Can you work these out from the model? Positions are in its coordinate system, mm. A direction names the side the tool comes from. Round coordinates to 2 decimals unless told otherwise and drop trailing zeros. Write each loop counter-clockwise with the first axis right and the second up, starting at its lowest first coordinate (ties: lowest second). Pieces come first, ordered by that corner, then holes. Notation, with made-up numbers: M -16.75,-35 L 5.25,-35 A17 ccw 5.25,-20 Z; hole C 34,65 d11. An arc over 180 degrees is marked long. Answer in a Markdown table with one row per item. Add a question column.
(1) If I drill on probe 1 along Z at (x, y) = (-1.25, 12.5); probe 2 along Y at (x, z) = (7.5, 1.7); probe 3 along X at (y, z) = (11.25, 166), over which ranges is the centre line in solid material (lowest first)?
(2) I'm going to push flat-ended pins straight in: pin 1 (2.5 mm diameter, centred on x = 16.5, z = 139.5, fed in from -Y); pin 2 (2 mm diameter, centred on y = 12.4, z = 100, fed in from +X); pin 3 (6.5 mm diameter, centred on x = 10, y = 7, fed in from +Z); pin 4 (4 mm diameter, centred on x = 3.5, y = 17, fed in from +Z). Where does each tip first touch, or does it pass through?
(3) If we mould it in two halves opening along X, with no side actions, what happens to faces 6 (the face through (9.885, -1.846, 1.521)), 7 (the face through (18, 10, 114)), 8 (the face through (7, 6, 3)), 9 (the face through (7, 19.403, 116))? For each: released by +X, released by -X, zero draft, split by the parting line, or undercut.
(4) Suppose I cut it at A-A, the plane y = 7.25. Write out the boundary of the cut face in (x, z).
(5) Suppose I cut it at B-B, the plane z = 135. Write out the boundary of the cut face in (x, y).
(6) For faces 1 (the face through (-1, 11, 8)), 2 (the face through (9, 20, 224)), 3 (the face through (7.17, 20.88, 220.48)), 4 (the face through (16, 11, 8)), 5 (the face through (0, 8, 114)), which set-ups out of +Z, -Z, +X, -X, +Y, -Y let a thin tool reach every point of the face, with its end or its side?
from build123d import *

# Parameters (mm, degrees)
F1_DEPTH  = 15
F2_W      = 3
F2_H      = 216
F3_DEPTH  = 25
F4_R      = 2.5
F5_DEPTH  = 3
F6_W      = 1
F6_H      = 0.5
F7_DEPTH  = 3
F8_R      = 1
F9_R      = 2.5
F9_R_2    = 1.2
F10_DEPTH = 3
F11_R     = 1.2
F12_DEPTH = 34.2
F13_DEPTH = 3
F14_R     = 2


with BuildPart() as f1:
    # F0 (on Right) → F1 (new body)
    with BuildSketch(Plane.YZ):
        Polygon((-7.5968508422, 3), (-7.5968508422, 0), (22.4031491578, 0), (22.4031491578, 224), (19.4031491578, 224), (19.4031491578, 3), align=None)
    extrude(amount=F1_DEPTH)

    # F2 (on face) → F3 (join)
    with BuildSketch(Plane(origin=(0, 22.4031491578, 0), x_dir=(-1, 0, 0), z_dir=(0, 1, 0))):
        with Locations((1.5, 116)):
            Rectangle(F2_W, F2_H)
        with Locations((-16.5, 116)):
            Rectangle(F2_W, F2_H)
    extrude(amount=-F3_DEPTH)

    # F4 (on face) → F5 (cut)
    with BuildSketch(Plane.XY.offset(3)):
        with Locations((7.5, -2.5968508422)):
            Circle(F4_R)
        with Locations((7.5, 12.4031491578)):
            Circle(F4_R)
    extrude(amount=-F5_DEPTH, mode=Mode.SUBTRACT)

    # F6 (on face) → F7 (cut)
    with BuildSketch(Plane.XZ.offset(-19.4031491578)):
        with Locations((0.5, 7.75)):
            Rectangle(F6_W, F6_H)
        with Locations((14.5, 7.75)):
            Rectangle(F6_W, F6_H)
    extrude(amount=-F7_DEPTH, mode=Mode.SUBTRACT)

    # F8
    f8_edges = [f1.edges().sort_by_distance(p)[0] for p in [
        (7.5, 19.403149, 3),
        (7.5, 22.403149, 0),
        (0, 19.403149, 116),
        (-3, 22.403149, 116),
        (18, 22.403149, 116),
        (15, 19.403149, 116),
    ]]
    fillet(f8_edges, radius=F8_R)

    # F9 (on face) → F10 (cut)
    with BuildSketch(Plane.XZ.offset(-19.4031491578)):
        with Locations((7.5, 218)):
            Circle(F9_R)
        with Locations((7.5, 100)):
            Circle(F9_R_2)
        with Locations((7.5, 200)):
            Circle(F9_R_2)
    extrude(amount=-F10_DEPTH, mode=Mode.SUBTRACT)

    # F11 (on face) → F12 (cut)
    with BuildSketch(Plane(origin=(-3, 0, 0), x_dir=(0, -1, 0), z_dir=(-1, 0, 0))):
        with Locations((-12.4031491578, 200)):
            Circle(F11_R)
        with Locations((-12.4031491578, 100)):
            Circle(F11_R)
    extrude(amount=-F12_DEPTH, mode=Mode.SUBTRACT)

    # F13 (add, symmetric): faces of the model
    f13_faces = [f1.faces().sort_by_distance(p)[0] for p in [
        (0, 9.1577983799, 1.9953507779),
        (15, 9.1577983799, 1.9953507779),
    ]]
    extrude(f13_faces, amount=F13_DEPTH, both=True, dir=(-1, 0, 0))

    # F14
    f14_edges = [f1.edges().sort_by_distance(p)[0] for p in [
        (-3, -7.596851, 1.5),
        (18, -7.596851, 1.5),
        (-1.5, -2.596851, 8),
        (16.5, -2.596851, 8),
        (-1.5, -2.596851, 224),
        (16.5, -2.596851, 224),
    ]]
    fillet(f14_edges, radius=F14_R)


solid = f1.part
Calculated:
| question | item | result |
|---|---|---|
| 1 | probe 1 | 0 to 3, 8 to 98.8, 101.2 to 198.8, 201.2 to 224 |
| 1 | probe 2 | -7.6 to -5.1, -0.1 to 9.9, 14.9 to 22.4 |
| 1 | probe 3 | -3 to 0, 15 to 18 |
| 2 | pin 1 | y = -2.6 |
| 2 | pin 2 | through |
| 2 | pin 3 | z = 3 |
| 2 | pin 4 | z = 3.2 |
| 3 | face 6 | undercut |
| 3 | face 7 | released by +X |
| 3 | face 8 | zero draft |
| 3 | face 9 | undercut |
| 4 | outline | M -3,0 L 18,0 L 18,3 L -3,3 Z; M -3,8 L 0,8 L 0,224 L -3,224 Z; M 15,8 L 18,8 L 18,224 L 15,224 Z |
| 5 | outline | M -3,-2.6 L 0,-2.6 L 0,18.4 A1 cw 1,19.4 L 14,19.4 A1 cw 15,18.4 L 15,-2.6 L 18,-2.6 L 18,21.4 A1 ccw 17,22.4 L -2,22.4 A1 ccw -3,21.4 Z |
| 6 | face 1 | -X, +Y, -Y |
| 6 | face 2 | +Z, +X, -X, +Y, -Y |
| 6 | face 3 | +Y, -Y |
| 6 | face 4 | +X, +Y, -Y |
| 6 | face 5 | +Z, -Y |
